Design review of the part built by this model. Coordinates are the model's own, in mm. Face numbers are marked on the shaded views. A direction names the side the tool comes from. Round coordinates to 2 decimals unless told otherwise and drop trailing zeros. Order: outer loops, then holes, each group sorted by start corner. A loop starts at its lowest first (then second) coordinate and runs counter-clockwise, first axis right, second up. Notation, with made-up numbers: M -11,-14.5 L 33,-14.5 A18 ccw 33,10.5 Z; hole C 18.25,23.5 d4. An arc over 180 degrees is marked long. Write each question's results on one line, items separated by ' | '. Start each with the question number.
Item 1: Machinability: for the marked faces 4, 5 and 6, which of the approach directions +Z, -Z, +X, -X, +Y, -Y give a long, thin tool a straight path to every point of the face, cutting with its end or side? Answer none if there is none.
Item 2: Wall thickness on line 1 (Z direction, x = 25.4, y = 3); line 2 (X direction, y = -2, z = 7.5); line 3 (Y direction, x = 21, z = -27): over which ranges is each line inside the solid? List them lowest first. Write a range as [from, to].
Item 3: The part is to be moulded in two halves that separate along X. For the marked faces 1, 2 and 3, say which applies: +X half, -X half, draft (parallel to the pull), parting line (faces both ways), or undercut.
Item 4: Take a section at B-B, the plane x = 7.5. Write out the cut boundary in (y, z).
Item 5: Take a section at D-D, the plane z = -14. Write out the cut boundary in (x, y).
Item 6: Take a section at A-A, the plane y = -7. Write out the cut boundary in (x, z), plus the area to 3 significant figures.
Item 7: Clearance check with flat-ended pins moving along their axes: pin 1 (2.5 mm diameter, centred on x = 43.5, y = -6, fed in from -Z); pin 2 (2.5 mm diameter, centred on x = 26, z = -6.5, fed in from +Y); pin 3 (10 mm diameter, centred on y = -4, z = -24, fed in from -X); pin 4 (3 mm diameter, centred on x = 34.5, y = 8, fed in from -Z). State where each tip first meets the part, or that it passes through.
Item 8: Take a section at C-C, the plane y = 2.25. Write out the cut boundary in (x, z).
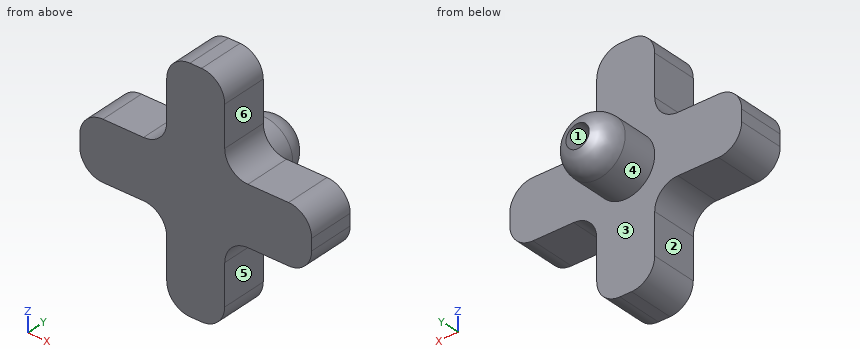
```python
from build123d import *

# Parameters (mm, degrees)
F0_W     = 19.05
F0_H     = 12.7
F0_W_2   = 12.7
F0_H_2   = 19.05
F1_DEPTH = 10.16
F2_R     = 5.08
F3_R     = 6.35
F3_R_2   = 2.54
F4_DEPTH = 12.7
F5_DEPTH = 2.54


# Not quite as in the source:
# - a fillet or chamfer that OpenCascade refuses, or shapes differently, is made with other operations: its cross-section is extruded or revolved along the edge and cut away or added


with BuildPart() as f1:
    # F0 (on Front) → F1 (new body)
    with BuildSketch(Plane.XZ):
        with Locations((9.525, -6.35)):
            Rectangle(F0_W, F0_H)
        with Locations((25.4, 9.525)):
            Rectangle(F0_W_2, F0_H_2)
        with Locations((25.4, -6.35)):
            Rectangle(F0_W_2, F0_H)
        with Locations((41.275, -6.35)):
            Rectangle(F0_W, F0_H)
        with Locations((25.4, -22.225)):
            Rectangle(F0_W_2, F0_H_2)
    extrude(amount=F1_DEPTH)

    # F2
    f2_edges = [f1.edges().sort_by_distance(p)[0] for p in [
        (19.05, -5.08, -12.7),
        (19.05, -5.08, 0),
        (31.75, -5.08, 0),
        (31.75, -5.08, -12.7),
        (0, -5.08, 0),
        (0, -5.08, -12.7),
        (19.05, -5.08, -31.75),
        (31.75, -5.08, -31.75),
        (50.8, -5.08, -12.7),
        (50.8, -5.08, 0),
        (31.75, -5.08, 19.05),
        (19.05, -5.08, 19.05),
    ]]
    fillet(f2_edges, radius=F2_R)

    # F3 (on face) → F4 (join)
    with BuildSketch(Plane(origin=(0, 0, 0), x_dir=(-1, 0, 0), z_dir=(0, 1, 0))):
        with Locations((-25.4, -6.35)):
            Circle(F3_R)
        with Locations((-25.4, -6.35)):
            Circle(F3_R_2, mode=Mode.SUBTRACT)
    extrude(amount=F4_DEPTH)

    # F5 (cut): a face of the model
    f5_faces = [f1.faces().sort_by_distance(p)[0] for p in [
        (25.4, 0, -6.35),
    ]]
    extrude(f5_faces, amount=-F5_DEPTH, mode=Mode.SUBTRACT)

    # F6: fillet of radius 5.08 on 1 edges, made by hand

    # F6_s1 → F6_t2 (revolve, cut)
    with BuildSketch(Plane.XY.offset(-6.35)):
        with BuildLine():
            ThreePointArc((19.05, 7.7813111503), (20.1139073716, 10.8921631237), (22.86, 12.7))
            Line((22.86, 12.7), (19.05, 12.7))
            Line((19.05, 12.7), (19.05, 7.7813111503))
        make_face()
    revolve(axis=Axis((25.4, 12.7, -6.35), (0, 1, 0)), mode=Mode.SUBTRACT)


solid = f1.part
```
Results list:
1) face 4: +Y | face 5: -Z, +X, +Y, -Y | face 6: +Z, +X, +Y, -Y
2) line 1: [-12.7, -8.89], [-3.81, 0] | line 2: [19.05, 31.75] | line 3: [-10.16, 0]
3) face 1: undercut | face 2: -X half | face 3: draft
4) outline: M -10.16,-12.7 L 0,-12.7 L 0,0 L -10.16,0 Z
5) outline: M 17.36,-10.16 L 33.44,-10.16 L 33.44,0 L 17.36,0 Z
6) outline: M 0,-7.62 A5.08 ccw 5.08,-12.7 L 13.97,-12.7 A5.08 cw 19.05,-17.78 L 19.05,-26.67 A5.08 ccw 24.13,-31.75 L 26.67,-31.75 A5.08 ccw 31.75,-26.67 L 31.75,-17.78 A5.08 cw 36.83,-12.7 L 45.72,-12.7 A5.08 ccw 50.8,-7.62 L 50.8,-5.08 A5.08 ccw 45.72,0 L 36.83,0 A5.08 cw 31.75,5.08 L 31.75,13.97 A5.08 ccw 26.67,19.05 L 24.13,19.05 A5.08 ccw 19.05,13.97 L 19.05,5.08 A5.08 cw 13.97,0 L 5.08,0 A5.08 ccw 0,-5.08 Z | area: 1,110 mm²
7) pin 1: z = -12.7 | pin 2: y = -2.54 | pin 3: x = 19.05 | pin 4: through
8) outline: C 25.4,-6.35 d12.7; hole C 25.4,-6.35 d5.08
